Verification items for the finished model (mm, model axes). A direction names the side the tool comes from. Coordinates: 2 decimals unless noted, no trailing zeros. Order: outer loops, then holes, each group sorted by start corner. A loop starts at its lowest first (then second) coordinate and runs counter-clockwise, first axis right, second up. Notation, with made-up numbers: (75, 11) -> (112, 11) arc R17 cw to (112, 34) -> close; hole circle Ø5 at (10, -38.75). An arc over 180 degrees is marked (long way). Write item = value, one per line. Start each with the question number.
1. Set-up check for faces 4 (the cylindrical face through (-25.044, 58.413, -0.335)), 5 (the flat face through (0, 45, 3)): record each of +Z, -Z, +X, -X, +Y, -Y from which the full face is reachable in a straight line by a thin tool's end or side.
2. Thickness scan on line 1 along Y through (x, z) = (-41, 0); line 2 along Z through (x, y) = (-35, 0); line 3 along Y through (x, z) = (-16, -5.75). Record the ranges inside material, lowest first. Write a range as from..to.
3. Cross-section at A-A on z = 0. Record the cut outline in (x, y), plus the area to 3 significant figures.
4. Cross-section at B-B on x = -5. Record the cut outline in (y, z), plus the area to 3 significant figures.
5. Cross-section at C-C on x = -58.5. Give the number of separate pieces and of enclosed holes in the cut face, plus the area to 3 significant figures.
6. Go/stop test with flat-tipped pins: P1, Ø1.5, axis at x = -43, y = 6, coming from the -Z side; P2, Ø3, axis at x = -60.5, z = -0.5, coming from the -Y side; P3, Ø1.5, axis at x = -56, z = -4, coming from the +Y side; P4, Ø4, axis at x = -63, y = 5.5, coming from the +Z side. Record where each tip stops, or that it passes through.
7. Release check for a two-part mould opening along Z. For faces 1 (the cylindrical face through (-25.76, -1.38, 6.2)), 2 (the flat face through (0, -6, -3)), 3 (the cylindrical face through (-25.76, -1.65, 7.44)) record: +Z half, -Z half, draft (parallel to the pull), parting line (faces both ways), or undercut.
from build123d import *

# Parameters (mm, degrees)
F1_R   = 7.62
F1_R_2 = 6.35


with BuildPart() as f2:
    # F2: sweep along a path in F0
    with BuildLine(Plane.XY) as f2_path:
        Line((0, 0), (-50.8, 0))
        ThreePointArc((-50.8, 0), (-76.2, 25.4), (-50.8, 50.8))
        Line((-50.8, 50.8), (0, 50.8))
    # F1 (on Right) → F2 (sweep)
    with BuildSketch(Plane.YZ):
        Circle(F1_R)
        Circle(F1_R_2, mode=Mode.SUBTRACT)
    sweep(path=f2_path.line)


solid = f2.part
Worked out:
q1.face_4 = +X
q1.face_5 = +Z, -Z, +X, +Y, -Y
q2.line_1 = -7.62..-6.35, 6.35..7.62, 43.18..44.45, 57.15..58.42
q2.line_2 = -7.62..-6.35, 6.35..7.62
q2.line_3 = -5..-2.69, 2.69..5, 45.8..48.11, 53.49..55.8
q3.outline = (-50.8, -7.62) -> (0, -7.62) -> (0, -6.35) -> (-50.8, -6.35) arc R31.75 cw to (-50.8, 57.15) -> (0, 57.15) -> (0, 58.42) -> (-50.8, 58.42) arc R33.02 ccw to start; (-50.8, 6.35) -> (0, 6.35) -> (0, 7.62) -> (-50.8, 7.62) arc R17.78 cw to (-50.8, 43.18) -> (0, 43.18) -> (0, 44.45) -> (-50.8, 44.45) arc R19.05 ccw to start
q3.area = 461 mm²
q4.outline = circle Ø15.24 at (0, 0); circle Ø15.24 at (50.8, 0); hole circle Ø12.7 at (0, 0); hole circle Ø12.7 at (50.8, 0)
q4.area = 111 mm²
q5.separate_pieces = 2
q5.enclosed_holes = 2
q5.area = 118 mm²
q6.P1 = -5.52
q6.P2 = -6.58
q6.P3 = 57.29
q6.P4 = 7.62
q7.face_1 = undercut
q7.face_2 = draft
q7.face_3 = parting line
